from build123d import *

# Parameters (mm, degrees)
SKETCH1_R           = 0.75
BOSS_EXTRUDE1_DEPTH = 2.7


with BuildPart() as part:
    # Sketch1 → Boss-Extrude1 (new body)
    with BuildSketch(Plane.XY):
        Polygon((-30.072121707, -52.412620775), (-30.072121707, 54.887379225), (29.927878293, 54.887379225), (29.927878293, -52.412620775), (17.927878293, -52.412620775), (17.927878293, -55.112620775), (5.927878293, -55.112620775), (5.927878293, -52.412620775), (-6.072121707, -52.412620775), (-6.072121707, -55.112620775), (-18.072121707, -55.112620775), (-18.072121707, -52.412620775), align=None)
        with Locations((-8.543810279, 48.617379225)):
            Circle(SKETCH1_R, mode=Mode.SUBTRACT)
        with Locations((-8.543810279, 7.977379225)):
            Circle(SKETCH1_R, mode=Mode.SUBTRACT)
        with Locations((-23.783810279, 7.977379225)):
            Circle(SKETCH1_R, mode=Mode.SUBTRACT)
        with Locations((-23.783810279, 48.617379225)):
            Circle(SKETCH1_R, mode=Mode.SUBTRACT)
        with Locations((23.676189721, 48.617379225)):
            Circle(SKETCH1_R, mode=Mode.SUBTRACT)
        with Locations((23.676189721, 7.977379225)):
            Circle(SKETCH1_R, mode=Mode.SUBTRACT)
        with Locations((8.436189721, 7.977379225)):
            Circle(SKETCH1_R, mode=Mode.SUBTRACT)
        with Locations((8.436189721, 48.617379225)):
            Circle(SKETCH1_R, mode=Mode.SUBTRACT)
        with BuildLine():
            Line((-10.697202951, 49.887379225), (-21.630417607, 49.887379225))
            ThreePointArc((-21.630417607, 49.887379225), (-22.023594521, 46.842093195), (-25.072121707, 46.474891496))
            Line((-25.072121707, 46.474891496), (-25.072121707, 10.119866953))
            ThreePointArc((-25.072121707, 10.119866953), (-22.023594521, 9.752665254), (-21.630417607, 6.707379225))
            Line((-21.630417607, 6.707379225), (-10.697202951, 6.707379225))
            ThreePointArc((-10.697202951, 6.707379225), (-10.319058772, 9.73763284), (-7.292121707, 10.141466958))
            Line((-7.292121707, 10.141466958), (-7.292121707, 46.453291491))
            ThreePointArc((-7.292121707, 46.453291491), (-10.319058772, 46.85712561), (-10.697202951, 49.887379225))
        make_face(mode=Mode.SUBTRACT)
        with BuildLine():
            Line((21.522797049, 49.887379225), (10.589582393, 49.887379225))
            ThreePointArc((10.589582393, 49.887379225), (10.196405479, 46.842093195), (7.147878293, 46.474891496))
            Line((7.147878293, 46.474891496), (7.147878293, 10.119866953))
            ThreePointArc((7.147878293, 10.119866953), (10.196405479, 9.752665254), (10.589582393, 6.707379225))
            Line((10.589582393, 6.707379225), (21.522797049, 6.707379225))
            ThreePointArc((21.522797049, 6.707379225), (21.900941228, 9.73763284), (24.927878293, 10.141466958))
            Line((24.927878293, 10.141466958), (24.927878293, 46.453291491))
            ThreePointArc((24.927878293, 46.453291491), (21.900941228, 46.85712561), (21.522797049, 49.887379225))
        make_face(mode=Mode.SUBTRACT)
    extrude(amount=BOSS_EXTRUDE1_DEPTH)


solid = part.part
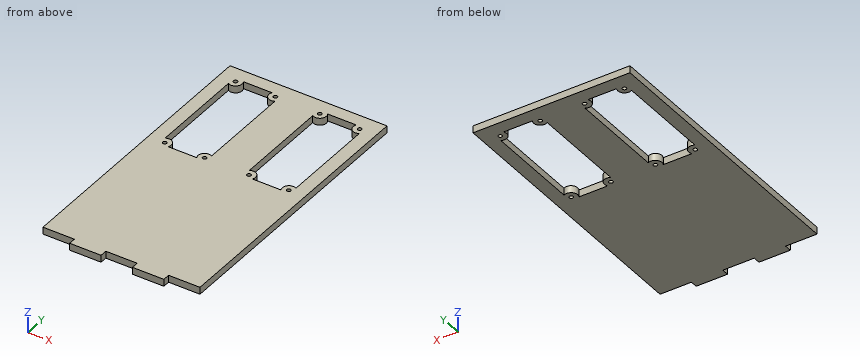
Here's how the part is built. I have some questions about the finished solid (model axes, mm). Coordinates: 2 decimals unless noted, no trailing zeros. Order: outer loops, then holes, each group sorted by start corner. A loop starts at its lowest first (then second) coordinate and runs counter-clockwise, first axis right, second up. Notation, with made-up numbers: (89.25, -29) -> (114.25, -29) arc R35 cw to (114.25, 3) -> close; hole circle Ø2 at (-15.75, 57.25). An arc over 180 degrees is marked (long way). Answer in a Markdown table with one row per item.
(1) I want a section at C-C on z = 1.85. Count the separate pieces of the cut face and the enclosed holes in it, then the cut area to 3 significant figures.
Answer key:
| item | result |
|---|---|
| separate pieces | 1 |
| enclosed holes | 10 |
| area | 5,050 mm^2 |
(2) Will these pins go through, and if not, where does the flat tip stop? pin 1 Ø0.9 at (x, y) = (-23.78, 48.62) entering from +Z; pin 2 Ø0.8 at (x, z) = (-0.5, 1.5) entering from -Y; pin 3 Ø1.5 at (x, y) = (7, 29) entering from -Z; pin 4 Ø1.4 at (y, z) = (-54.5, 1.5) entering from +X.
Answer key:
| item | result |
|---|---|
| pin 1 | through |
| pin 2 | y = -52.41 |
| pin 3 | z = 0 |
| pin 4 | x = 17.93 |
(3) Please list where these lines run through material, in increasing order: probe 1 along X at (y, z) = (16.5, 1); probe 2 along Y at (x, z) = (-8.5, 1.5); probe 3 along Y at (x, z) = (9, 1.95).
Answer key:
| item | result |
|---|---|
| probe 1 | -30.07 to -25.07, -7.29 to 7.15, 24.93 to 29.93 |
| probe 2 | -55.11 to 7.23, 8.73 to 10.48, 46.12 to 47.87, 49.37 to 54.89 |
| probe 3 | -55.11 to 7.48, 8.47 to 10.41, 46.18 to 48.12, 49.11 to 54.89 |
(4) I want a section at A-A on y = 17.5. List the corners of the cut face in (x, z) for me, then the cut area to 3 significant figures.
Answer key:
| item | result |
|---|---|
| outline | (-30.07, 0) -> (-25.07, 0) -> (-25.07, 2.7) -> (-30.07, 2.7) -> close; (-7.29, 0) -> (7.15, 0) -> (7.15, 2.7) -> (-7.29, 2.7) -> close; (24.93, 0) -> (29.93, 0) -> (29.93, 2.7) -> (24.93, 2.7) -> close |
| area | 66.0 mm^2 |
(5) I want a section at B-B on x = -1.5. List the corners of the cut face in (y, z) for me.
Answer key:
| item | result |
|---|---|
| outline | (-52.41, 0) -> (54.89, 0) -> (54.89, 2.7) -> (-52.41, 2.7) -> close |
